```python
from build123d import *

# Parameters (mm, degrees)
F0_R     = 11.43
F1_DEPTH = 5.08
F2_R     = 5.07999
F3_R     = 8.89
F4_DEPTH = 18.288
F5_R     = 6.0681762548
F6_DEPTH = 12.7


# Not quite as in the source:
# - a fillet or chamfer is up to 0.001 mm smaller than in the source, because OpenCascade refuses the exact size


with BuildPart() as f1:
    # F0 (on Top) → F1 (new body)
    with BuildSketch(Plane.XY):
        Circle(F0_R)
    extrude(amount=F1_DEPTH)

    # F2 (radius 5.08 in the source; OpenCascade refuses exactly that, so slightly less here)
    f2_edges = [f1.edges().sort_by_distance(p)[0] for p in [
        (-11.43, 0, 5.08),
    ]]
    fillet(f2_edges, radius=F2_R)

    # F3 (on face) → F4 (join)
    with BuildSketch(Plane(origin=(0, 0, 0), x_dir=(1, 0, 0), z_dir=(0, 0, -1))):
        Circle(F3_R)
    extrude(amount=F4_DEPTH)

    # F5 (on face) → F6 (cut)
    with BuildSketch(Plane(origin=(0, 0, -18.288), x_dir=(1, 0, 0), z_dir=(0, 0, -1))):
        Circle(F5_R)
    extrude(amount=-F6_DEPTH, mode=Mode.SUBTRACT)


solid = f1.part
```
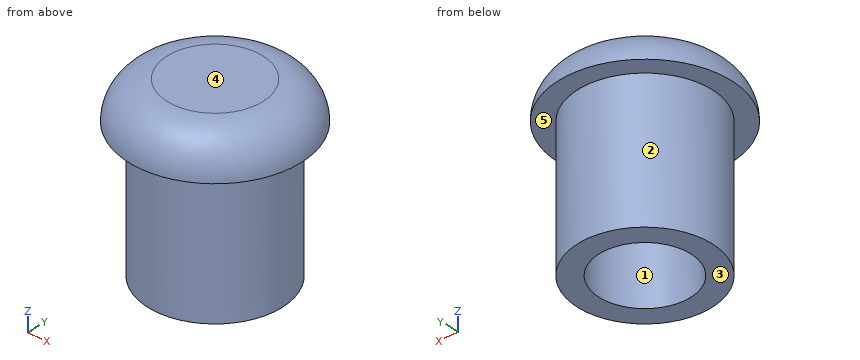
Geometry check sheet. Reference: the model listing, model coordinates, mm. Face numbers are marked on the shaded views. A direction names the side the tool comes from. Coordinates: 2 decimals unless noted, no trailing zeros. Order: outer loops, then holes, each group sorted by start corner. A loop starts at its lowest first (then second) coordinate and runs counter-clockwise, first axis right, second up. Notation, with made-up numbers: (19.5, 39) - (73.5, 39) arc R14 ccw to (73.5, 56) - close; hole circle Ø10 at (40, -16.75). An arc over 180 degrees is marked (long way). Answer in a Markdown table with one row per item. Add a question column.
1. Material ranges on L1, parallel to Y at x = 0, z = -9; L2, parallel to Z at x = 1.75, y = 1.25; L3, parallel to Y at x = -3.5, z = -8, recorded low to high. Write a range as [from, to].
2. Section check D-D (z = -2.5). Enter the section's corners in (x, y), plus the area to 3 significant figures.
3. Draft check along Y on the marked faces 1, 2 and 3. Enter one of: +Y half, -Y half, draft (parallel to the pull), parting line (faces both ways), or undercut.
4. Gauge pin test, flat ends, axial feed: pin 1 Ø1 at (x, z) = (-3.5, -7.5) entering from -Y; pin 2 Ø2 at (x, y) = (-5.5, -8.5) entering from +Z; pin 3 Ø12 at (x, z) = (7.5, 0) entering from -Y. Record the tip position at first contact, or that the pin passes through.
5. Access from +Z, -Z, +X, -X, +Y, -Y to the whole of each face (thin tool, end or side, straight path). Record for the marked faces 4 and 5.
6. Section check B-B (z = -7.25). Enter the section's corners in (x, y).
Data:
| question | item | result |
|---|---|---|
| 1 | L1 | y = [-8.89, -6.07], [6.07, 8.89] |
| 1 | L2 | z = [-5.59, 5.08] |
| 1 | L3 | y = [-8.17, -4.96], [4.96, 8.17] |
| 2 | outline | circle Ø17.78 at (0, 0) |
| 2 | area | 248 mm² |
| 3 | face 1 | undercut |
| 3 | face 2 | parting line |
| 3 | face 3 | draft |
| 4 | pin 1 | stops at y = -8.37 |
| 4 | pin 2 | stops at z = 4.26 |
| 4 | pin 3 | stops at y = -11.33 |
| 5 | face 4 | +Z, +X, -X, +Y, -Y |
| 5 | face 5 | -Z |
| 6 | outline | circle Ø17.78 at (0, 0); hole circle Ø12.14 at (0, 0) |
